Design review of the part built by this model. Coordinates are the model's own, in mm. Give positions to 0.01 mm unless a question says otherwise; leave off trailing zeros. Loops run counter-clockwise (first coordinate to the right, second up) from the corner with the lowest first, then second, coordinate; pieces in that order, holes last. Notation, with made-up numbers: (29, 74) - (64, 74) arc R17 ccw to (64, 103) - close; hole circle Ø5 at (38.5, -28.5). An arc over 180 degrees is marked (long way). One line per item, written item: value. Start each with the question number.
```python
from build123d import *

# Parameters (mm, degrees)
SKETCH1_W           = 260
SKETCH1_H           = 600
SKETCH1_R           = 2
SKETCH1_R_2         = 1.6
SKETCH1_W_2         = 100
SKETCH1_H_2         = 320
BOSS_EXTRUDE1_DEPTH = 3.175
FILLET1_R           = 3


with BuildPart() as part:
    # Sketch1 → Boss-Extrude1 (new body)
    with BuildSketch(Plane(origin=(0, 0, 0), x_dir=(1, 0, 0), z_dir=(0, 1, 0))):
        Rectangle(SKETCH1_W, SKETCH1_H)
        with Locations(Location((120, 290, 0), (0, 0, 270))):
            Circle(SKETCH1_R, mode=Mode.SUBTRACT)
        with Locations(Location((120, 232, 0), (0, 0, 270))):
            Circle(SKETCH1_R, mode=Mode.SUBTRACT)
        with Locations(Location((120, 174, 0), (0, 0, 270))):
            Circle(SKETCH1_R, mode=Mode.SUBTRACT)
        with Locations(Location((120, 116, 0), (0, 0, 270))):
            Circle(SKETCH1_R, mode=Mode.SUBTRACT)
        with Locations(Location((120, 58, 0), (0, 0, 270))):
            Circle(SKETCH1_R, mode=Mode.SUBTRACT)
        with Locations(Location((120, 0, 0), (0, 0, 270))):
            Circle(SKETCH1_R, mode=Mode.SUBTRACT)
        with Locations(Location((120, -58, 0), (0, 0, 270))):
            Circle(SKETCH1_R, mode=Mode.SUBTRACT)
        with Locations(Location((120, -116, 0), (0, 0, 270))):
            Circle(SKETCH1_R, mode=Mode.SUBTRACT)
        with Locations(Location((120, -174, 0), (0, 0, 270))):
            Circle(SKETCH1_R, mode=Mode.SUBTRACT)
        with Locations(Location((120, -232, 0), (0, 0, 270))):
            Circle(SKETCH1_R, mode=Mode.SUBTRACT)
        with Locations(Location((120, -290, 0), (0, 0, 270))):
            Circle(SKETCH1_R, mode=Mode.SUBTRACT)
        with Locations(Location((-120, 232, 0), (0, 0, 90))):
            Circle(SKETCH1_R, mode=Mode.SUBTRACT)
        with Locations(Location((-120, -290, 0), (0, 0, 90))):
            Circle(SKETCH1_R, mode=Mode.SUBTRACT)
        with Locations(Location((-120, -232, 0), (0, 0, 90))):
            Circle(SKETCH1_R, mode=Mode.SUBTRACT)
        with Locations(Location((-120, -174, 0), (0, 0, 90))):
            Circle(SKETCH1_R, mode=Mode.SUBTRACT)
        with Locations(Location((-120, -116, 0), (0, 0, 90))):
            Circle(SKETCH1_R, mode=Mode.SUBTRACT)
        with Locations(Location((-120, -58, 0), (0, 0, 90))):
            Circle(SKETCH1_R, mode=Mode.SUBTRACT)
        with Locations(Location((-120, 0, 0), (0, 0, 90))):
            Circle(SKETCH1_R, mode=Mode.SUBTRACT)
        with Locations(Location((-120, 58, 0), (0, 0, 90))):
            Circle(SKETCH1_R, mode=Mode.SUBTRACT)
        with Locations(Location((-120, 116, 0), (0, 0, 90))):
            Circle(SKETCH1_R, mode=Mode.SUBTRACT)
        with Locations(Location((-120, 174, 0), (0, 0, 90))):
            Circle(SKETCH1_R, mode=Mode.SUBTRACT)
        with Locations(Location((-120, 290, 0), (0, 0, 90))):
            Circle(SKETCH1_R, mode=Mode.SUBTRACT)
        with Locations(Location((112, 235, 0), (0, 0, 270))):
            Circle(SKETCH1_R_2, mode=Mode.SUBTRACT)
        with Locations(Location((-112, 235, 0), (0, 0, 90))):
            Circle(SKETCH1_R_2, mode=Mode.SUBTRACT)
        with Locations(Location((112, -235, 0), (0, 0, 90))):
            Circle(SKETCH1_R_2, mode=Mode.SUBTRACT)
        with Locations(Location((-112, -235, 0), (0, 0, 270))):
            Circle(SKETCH1_R_2, mode=Mode.SUBTRACT)
        with Locations(Location((104, 290, 0), (0, 0, 270))):
            Circle(SKETCH1_R, mode=Mode.SUBTRACT)
        with Locations(Location((104, 232, 0), (0, 0, 270))):
            Circle(SKETCH1_R, mode=Mode.SUBTRACT)
        with Locations(Location((104, 174, 0), (0, 0, 270))):
            Circle(SKETCH1_R, mode=Mode.SUBTRACT)
        with Locations(Location((104, 116, 0), (0, 0, 270))):
            Circle(SKETCH1_R, mode=Mode.SUBTRACT)
        with Locations(Location((104, 58, 0), (0, 0, 270))):
            Circle(SKETCH1_R, mode=Mode.SUBTRACT)
        with Locations(Location((104, 0, 0), (0, 0, 270))):
            Circle(SKETCH1_R, mode=Mode.SUBTRACT)
        with Locations(Location((104, -58, 0), (0, 0, 270))):
            Circle(SKETCH1_R, mode=Mode.SUBTRACT)
        with Locations(Location((104, -116, 0), (0, 0, 270))):
            Circle(SKETCH1_R, mode=Mode.SUBTRACT)
        with Locations(Location((104, -174, 0), (0, 0, 270))):
            Circle(SKETCH1_R, mode=Mode.SUBTRACT)
        with Locations(Location((104, -232, 0), (0, 0, 270))):
            Circle(SKETCH1_R, mode=Mode.SUBTRACT)
        with Locations(Location((104, -290, 0), (0, 0, 270))):
            Circle(SKETCH1_R, mode=Mode.SUBTRACT)
        with Locations(Location((-104, -290, 0), (0, 0, 90))):
            Circle(SKETCH1_R, mode=Mode.SUBTRACT)
        with Locations(Location((-104, -174, 0), (0, 0, 90))):
            Circle(SKETCH1_R, mode=Mode.SUBTRACT)
        with Locations(Location((-104, -116, 0), (0, 0, 90))):
            Circle(SKETCH1_R, mode=Mode.SUBTRACT)
        with Locations(Location((-104, -58, 0), (0, 0, 90))):
            Circle(SKETCH1_R, mode=Mode.SUBTRACT)
        with Locations(Location((-104, 0, 0), (0, 0, 90))):
            Circle(SKETCH1_R, mode=Mode.SUBTRACT)
        with Locations(Location((-104, 58, 0), (0, 0, 90))):
            Circle(SKETCH1_R, mode=Mode.SUBTRACT)
        with Locations(Location((-104, 116, 0), (0, 0, 90))):
            Circle(SKETCH1_R, mode=Mode.SUBTRACT)
        with Locations(Location((-104, 174, 0), (0, 0, 90))):
            Circle(SKETCH1_R, mode=Mode.SUBTRACT)
        with Locations(Location((-104, 232, 0), (0, 0, 90))):
            Circle(SKETCH1_R, mode=Mode.SUBTRACT)
        with Locations(Location((-104, 290, 0), (0, 0, 90))):
            Circle(SKETCH1_R, mode=Mode.SUBTRACT)
        with Locations(Location((-104, -232, 0), (0, 0, 90))):
            Circle(SKETCH1_R, mode=Mode.SUBTRACT)
        with Locations(Location((112, 0, 0), (0, 0, 270))):
            Circle(SKETCH1_R_2, mode=Mode.SUBTRACT)
        with Locations(Location((-112, 0, 0), (0, 0, 90))):
            Circle(SKETCH1_R_2, mode=Mode.SUBTRACT)
        with Locations(Location((-50, -290, 0), (0, 0, 270))):
            Circle(SKETCH1_R_2, mode=Mode.SUBTRACT)
        with Locations(Location((-50, -266, 0), (0, 0, 270))):
            Circle(SKETCH1_R_2, mode=Mode.SUBTRACT)
        with Locations(Location((50, -266, 0), (0, 0, 90))):
            Circle(SKETCH1_R_2, mode=Mode.SUBTRACT)
        with Locations(Location((50, -290, 0), (0, 0, 90))):
            Circle(SKETCH1_R_2, mode=Mode.SUBTRACT)
        with Locations(Location((-26, -290, 0), (0, 0, 90))):
            Circle(SKETCH1_R_2, mode=Mode.SUBTRACT)
        with Locations(Location((-26, -266, 0), (0, 0, 90))):
            Circle(SKETCH1_R_2, mode=Mode.SUBTRACT)
        with Locations(Location((26, -290, 0), (0, 0, 270))):
            Circle(SKETCH1_R_2, mode=Mode.SUBTRACT)
        with Locations(Location((26, -266, 0), (0, 0, 270))):
            Circle(SKETCH1_R_2, mode=Mode.SUBTRACT)
        with Locations(Location((-72, 290, 0), (0, 0, 90))):
            Circle(SKETCH1_R, mode=Mode.SUBTRACT)
        with Locations(Location((-72, 232, 0), (0, 0, 90))):
            Circle(SKETCH1_R, mode=Mode.SUBTRACT)
        with Locations(Location((-40, 290, 0), (0, 0, 90))):
            Circle(SKETCH1_R, mode=Mode.SUBTRACT)
        with Locations(Location((-40, 232, 0), (0, 0, 90))):
            Circle(SKETCH1_R, mode=Mode.SUBTRACT)
        with Locations(Location((-8, 290, 0), (0, 0, 90))):
            Circle(SKETCH1_R, mode=Mode.SUBTRACT)
        with Locations(Location((-8, 232, 0), (0, 0, 90))):
            Circle(SKETCH1_R, mode=Mode.SUBTRACT)
        with Locations(Location((24, 290, 0), (0, 0, 90))):
            Circle(SKETCH1_R, mode=Mode.SUBTRACT)
        with Locations(Location((24, 232, 0), (0, 0, 90))):
            Circle(SKETCH1_R, mode=Mode.SUBTRACT)
        with Locations(Location((56, 290, 0), (0, 0, 90))):
            Circle(SKETCH1_R, mode=Mode.SUBTRACT)
        with Locations(Location((56, 232, 0), (0, 0, 90))):
            Circle(SKETCH1_R, mode=Mode.SUBTRACT)
        with Locations(Location((88, 290, 0), (0, 0, 90))):
            Circle(SKETCH1_R, mode=Mode.SUBTRACT)
        with Locations(Location((88, 232, 0), (0, 0, 90))):
            Circle(SKETCH1_R, mode=Mode.SUBTRACT)
        with Locations(Location((-12, -251, 0), (0, 0, 270))):
            Circle(SKETCH1_R_2, mode=Mode.SUBTRACT)
        with Locations(Location((-2, -251, 0), (0, 0, 270))):
            Circle(SKETCH1_R_2, mode=Mode.SUBTRACT)
        with Locations(Location((-12, -211, 0), (0, 0, 90))):
            Circle(SKETCH1_R_2, mode=Mode.SUBTRACT)
        with Locations(Location((-2, -211, 0), (0, 0, 90))):
            Circle(SKETCH1_R_2, mode=Mode.SUBTRACT)
        with Locations((0, 40)):
            Rectangle(SKETCH1_W_2, SKETCH1_H_2, mode=Mode.SUBTRACT)
    extrude(amount=BOSS_EXTRUDE1_DEPTH)

    # Fillet1
    fillet1_edges = [part.edges().sort_by_distance(p)[0] for p in [
        (50, 1.5875, 120),
        (50, 1.5875, -200),
        (-50, 1.5875, -200),
        (-50, 1.5875, 120),
        (130, 1.5875, 300),
        (-130, 1.5875, 300),
        (-130, 1.5875, -300),
        (130, 1.5875, -300),
    ]]
    fillet(fillet1_edges, radius=FILLET1_R)


solid = part.part
```
(1) Take a section at C-C on y = 1.2. State how many separate pieces and enclosed holes the cut face has, and give its area (3 significant figures).
(2) For pin 1 Ø3 at (x, z) = (104, 116) entering from +Y; pin 2 Ø6.5 at (x, z) = (-104, 116) entering from -Y, all flat-tipped, find the tip position at first contact; note any pin that passes through.
(3) Take a section at B-B on z = -10. State the section outline as (x, y) points (3 decimals), and give its area (3 significant figures).
(4) Take a section at A-A on x = 39. State the section outline as (y, z) points (3 decimals).
(5) To check wall thickness, follow L1, parallel to X at y = 0.75, z = -58; L2, parallel to Z at x = 56, y = 2; L3, parallel to X at y = 1.9, z = 5. State the ranges of each line that lie inside material, in increasing order. Write a range as from..to.
Here are the results:
1. separate pieces: 1
1. enclosed holes: 75
1. area: 123,000 mm²
2. pin 1: through
2. pin 2: y = 0
3. outline: (-130, 0) - (-50, 0) - (-50, 3.175) - (-130, 3.175) - close; (50, 0) - (130, 0) - (130, 3.175) - (50, 3.175) - close
3. area: 508 mm²
4. outline: (0, -300) - (3.175, -300) - (3.175, -200) - (0, -200) - close; (0, 120) - (3.175, 120) - (3.175, 300) - (0, 300) - close
5. L1: -130..-122, -118..-106, -102..-50, 50..102, 106..118, 122..130
5. L2: -300..-292, -288..-234, -230..300
5. L3: -130..-50, 50..130
